```python
from build123d import *

# Parameters (mm, degrees)
SKETCH1_R           = 1.6
BOSS_EXTRUDE1_DEPTH = 1.2
FILLET1_R           = 1


with BuildPart() as part:
    # Sketch1 → Boss-Extrude1 (new body)
    with BuildSketch(Plane(origin=(0, 0, 0), x_dir=(1, 0, 0), z_dir=(0, 1, 0))):
        with BuildLine():
            Line((0, 0), (6.5, 0))
            ThreePointArc((6.5, 0), (5.914362684, 5.914362684), (0, 6.5))
            Line((0, 6.5), (0, 0))
        make_face()
        with Locations(Location((2.6, 2.6, 0), (0, 0, 270))):
            Circle(SKETCH1_R, mode=Mode.SUBTRACT)
    extrude(amount=BOSS_EXTRUDE1_DEPTH)

    # Fillet1
    fillet1_edges = [part.edges().sort_by_distance(p)[0] for p in [
        (0, 0.6, -6.5),
        (6.5, 0.6, 0),
        (0, 0.6, 0),
    ]]
    fillet(fillet1_edges, radius=FILLET1_R)


solid = part.part
```
Read the model definition and answer for the solid it produces. Units are mm, in the model's axes. Give positions to 0.01 mm unless a question says otherwise; leave off trailing zeros. Loops run counter-clockwise (first coordinate to the right, second up) from the corner with the lowest first, then second, coordinate; pieces in that order, holes last.
Item 1: The part is cut by section D-D (z = -5.5). Write down the section's boundary in (x, y), and give its area (3 significant figures).
Item 2: The part is cut by section A-A (x = 2.6). Write down the section's boundary in (y, z), and give its area (3 significant figures).
Item 3: This flat-tipped pin is pushed along its axis until it touches: pin 1 Ø3 at (x, z) = (5.5, -5.5) entering from -Y. Where does it stop, or does it pass through?
Item 4: The mould has two halves that part along X. Classify faces 1 (the flat face through (3, 1, 0)), 2 (the cylindrical face through (1.99, 0.59, -1.12)), 3 (the cylindrical face through (0.15, 0.61, -6.45)): released by +X, released by -X, zero draft, split by the parting line, or undercut.
Item 5: Find the intervals of material crossed by line 1 along X through (y, z) = (0.4, -2.6); line 2 along X through (y, z) = (0.15, -3.5); line 3 along Z through (x, y) = (2.5, 1.1), in increasing order.
Item 6: The part is cut by section C-C (y = 0.7). Write down the section's boundary in (x, z), and give its area (3 significant figures).
Item 7: The part is cut by section B-B (z = -2.6). Write down the section's boundary in (x, y), and give its area (3 significant figures).
Taken from the geometry:
1. outline: (0, 0) - (6.28, 0) - (6.28, 1.2) - (0, 1.2) - close
1. area: 7.54 mm2
2. outline: (0, -7.29) - (1.2, -7.29) - (1.2, -4.2) - (0, -4.2) - close; (0, -1) - (1.2, -1) - (1.2, 0) - (0, 0) - close
2. area: 4.90 mm2
3. pin 1: stops at y = 0
4. face 1: zero draft
4. face 2: undercut
4. face 3: released by -X
5. line 1: x = 0 to 1, 4.2 to 7.29
5. line 2: x = 0 to 1.28, 3.92 to 7.2
5. line 3: z = -7.29 to -4.2, -1 to 0
6. outline: (0, -5.92) arc R1 ccw to (0.57, -6.82) arc R4.69 ccw to (6.82, -0.57) arc R1 ccw to (5.92, 0) - (1, 0) arc R1 ccw to (0, -1) - close; hole circle Ø3.2 at (2.6, -2.6)
6. area: 38.7 mm2
7. outline: (0, 0) - (1, 0) - (1, 1.2) - (0, 1.2) - close; (4.2, 0) - (7.29, 0) - (7.29, 1.2) - (4.2, 1.2) - close
7. area: 4.90 mm2
